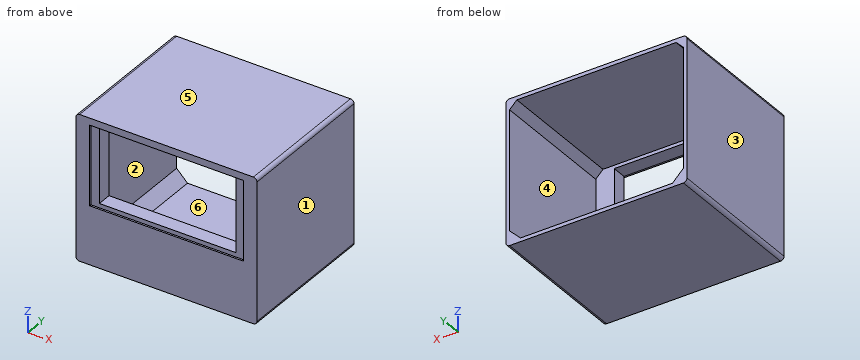
```python
from build123d import *

# Parameters (mm, degrees)
SKETCH1_W                 = 100
SKETCH1_H                 = 80
BOSS_EXTRUDE1_DEPTH       = 80.217571917
SHELL1_T                  = -2
SHELL1_THICKNESS_2_FACE_W = 76
SHELL1_THICKNESS_2_FACE_H = 96
SHELL1_THICKNESS_2_DEPTH  = 7
CUT_EXTRUDE2_DEPTH        = 180
FILLET3_R                 = 2
FILLET4_R                 = 2
CHAMFER2_SIZE             = 6
CHAMFER3_SIZE             = 6
CHAMFER4_SIZE             = 4
SKETCH4_W                 = 85
SKETCH4_H                 = 44
CUT_EXTRUDE3_DEPTH        = 1


with BuildPart() as part:
    # Sketch1 → Boss-Extrude1 (new body)
    with BuildSketch(Plane(origin=(0, 0, 0), x_dir=(1, 0, 0), z_dir=(0, 1, 0))):
        with Locations((9.074074074, -6.574074074)):
            Rectangle(SKETCH1_W, SKETCH1_H)
    extrude(amount=BOSS_EXTRUDE1_DEPTH)

    # Shell1
    shell1_openings = [part.faces().sort_by_distance(p)[0] for p in [
        (9.074074074, 80.217571917, 6.574074074),
    ]]
    offset(amount=SHELL1_T, openings=shell1_openings, kind=Kind.INTERSECTION)

    # Shell1 thickness 2 face (on inner face of the shell) → Shell1 thickness 2 (add)
    with BuildSketch(Plane(origin=(9.074074074, 2, 6.574074074), x_dir=(0, 0, -1), z_dir=(0, -1, 0))):
        Rectangle(SHELL1_THICKNESS_2_FACE_W, SHELL1_THICKNESS_2_FACE_H)
    extrude(amount=-SHELL1_THICKNESS_2_DEPTH)

    # Sketch3 → Cut-Extrude2 (cut)
    with BuildSketch(Plane(origin=(0, 80.217571917, 0), x_dir=(1, 0, 0), z_dir=(0, 1, 0))):
        Polygon((9.074074074, -1.163150467), (46.843833128, -1.163150467), (46.843833128, -42.758682986), (9.074074074, -42.758682986), (-28.653994459, -42.758682986), (-28.653994459, -1.163150467), align=None)
    extrude(amount=-CUT_EXTRUDE2_DEPTH, mode=Mode.SUBTRACT)

    # Fillet3
    fillet3_edges = [part.edges().sort_by_distance(p)[0] for p in [
        (-40.925925926, 40.108785958, 46.574074074),
    ]]
    fillet(fillet3_edges, radius=FILLET3_R)

    # Fillet4
    fillet4_edges = [part.edges().sort_by_distance(p)[0] for p in [
        (-40.925925926, 40.108785958, -33.425925926),
        (59.074074074, 40.108785958, -33.425925926),
        (59.074074074, 40.108785958, 46.574074074),
    ]]
    fillet(fillet4_edges, radius=FILLET4_R)

    # Chamfer2
    chamfer2_edges = [part.edges().sort_by_distance(p)[0] for p in [
        (-38.925925926, 44.608785958, -31.425925926),
    ]]
    chamfer(chamfer2_edges, length=CHAMFER2_SIZE)

    # Chamfer3
    chamfer3_edges = [part.edges().sort_by_distance(p)[0] for p in [
        (57.074074074, 44.608785958, -31.425925926),
    ]]
    chamfer(chamfer3_edges, length=CHAMFER3_SIZE)

    # Chamfer4
    chamfer4_edges = [part.edges().sort_by_distance(p)[0] for p in [
        (-38.925925926, 44.608785958, 44.574074074),
        (57.074074074, 44.608785958, 44.574074074),
    ]]
    chamfer(chamfer4_edges, length=CHAMFER4_SIZE)

    # Sketch4 → Cut-Extrude3 (cut)
    with BuildSketch(Plane.XZ):
        with Locations((9.08325413, 20.764850692)):
            Rectangle(SKETCH4_W, SKETCH4_H)
    extrude(amount=-CUT_EXTRUDE3_DEPTH, mode=Mode.SUBTRACT)


solid = part.part
```
Input: part model. Units: mm. Frame: model coordinates. Face numbers are marked on the shaded views. A direction names the side the tool comes from. Give positions to 0.01 mm unless a question says otherwise; leave off trailing zeros. Order: outer loops, then holes, each group sorted by start corner. A loop starts at its lowest first (then second) coordinate and runs counter-clockwise, first axis right, second up. Notation, with made-up numbers: M -7,62 L 34,62 A18 cw 34,70 Z; hole C 55.25,89 d6. An arc over 180 degrees is marked long. Return JSON: item names as keys, results as strings.
Item 1: Cut plane B-B (z = 26.5). Return loops of the section in (x, y).
Solutions:
{"outline": "M -40.93,0 L -33.42,0 L -33.42,1 L -28.65,1 L -28.65,9 L -38.93,9 L -38.93,80.22 L -40.93,80.22 Z; M 46.84,1 L 51.58,1 L 51.58,0 L 59.07,0 L 59.07,80.22 L 57.07,80.22 L 57.07,9 L 46.84,9 Z"}
Item 2: Cut plane C-C (y = 57). Return loops of the section in (x, z), then the cut area to 3 significant figures.
Solutions:
{"outline": "M -40.93,-31.43 A2 ccw -38.93,-33.43 L 57.07,-33.43 A2 ccw 59.07,-31.43 L 59.07,44.57 A2 ccw 57.07,46.57 L -38.93,46.57 A2 ccw -40.93,44.57 Z; hole M -38.93,-25.43 L -32.93,-31.43 L 51.07,-31.43 L 57.07,-25.43 L 57.07,40.57 L 53.07,44.57 L -34.93,44.57 L -38.93,40.57 Z", "area": "753 mm^2"}
Item 3: First-contact query: P1, Ø23, axis at x = -9.5, z = 7.5, coming from the +Y side. Flat tip, straight axial feed; report the tip coordinate or a pass-through.
Solutions:
{"P1": "y = 9"}
Item 4: Ray query, probe 1 along Z at (x, y) = (6, 31); probe 2 along X at (y, z) = (46.5, -25); probe 3 along Y at (x, z) = (-16, -29). Return the intervals inside material, ascending.
Solutions:
{"probe 1": "-33.43 to -31.43, 44.57 to 46.57", "probe 2": "-40.93 to -38.93, 57.07 to 59.07", "probe 3": "0 to 9"}
Item 5: Pull-direction query (Z, two-part tool) for the marked faces 3, 4, 5 and 6; classes: +Z half, -Z half, draft (parallel to the pull), parting line (faces both ways), or undercut.
Solutions:
{"face 3": "draft", "face 4": "undercut", "face 5": "+Z half", "face 6": "undercut"}
Item 6: Access query for the marked faces 1 and 2. Directions: +Z, -Z, +X, -X, +Y, -Y. A direction counts if a zero-diameter tool reaches every point of the face in a straight line with its end or side. Return the directions, or none.
Solutions:
{"face 1": "+Z, -Z, +X, +Y, -Y", "face 2": "+Y"}
